Design review of the part built by this model. Coordinates are the model's own, in mm. Round coordinates to 2 decimals unless told otherwise and drop trailing zeros. Order: outer loops, then holes, each group sorted by start corner. A loop starts at its lowest first (then second) coordinate and runs counter-clockwise, first axis right, second up.
from build123d import *

# Parameters (mm, degrees)
BOSS_EXTRUDE1_DEPTH = 15
FILLET1_R           = 10
FILLET2_R           = 10


with BuildPart() as part:
    # Sketch1 → Boss-Extrude1 (new body)
    with BuildSketch(Plane(origin=(0, 0, 0), x_dir=(0, 0, -1), z_dir=(1, 0, 0))):
        with BuildLine():
            Line((-62.5, 25), (-62.5, -87.5))
            Line((-62.5, -87.5), (62.5, -87.5))
            Line((62.5, -87.5), (62.5, 25))
            ThreePointArc((62.5, 25), (106.694173824, 131.694173824), (0, 87.5))
            ThreePointArc((0, 87.5), (-106.694173824, 131.694173824), (-62.5, 25))
        make_face()
    extrude(amount=BOSS_EXTRUDE1_DEPTH)

    # Fillet1
    fillet1_edges = [part.edges().sort_by_distance(p)[0] for p in [
        (7.5, 87.5, 0),
    ]]
    fillet(fillet1_edges, radius=FILLET1_R)

    # Fillet2
    fillet2_edges = [part.edges().sort_by_distance(p)[0] for p in [
        (7.5, -87.5, -62.5),
        (7.5, -87.5, 62.5),
    ]]
    fillet(fillet2_edges, radius=FILLET2_R)


solid = part.part
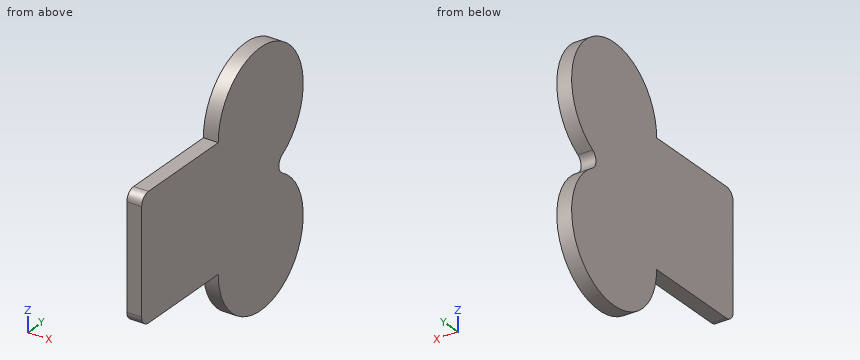
1) Take a section at C-C on z = 30.5. Give the boundary of the cut face in (x, y).
Results:
outline: (0, -87.5) - (15, -87.5) - (15, 141.19) - (0, 141.19) - close
2) To check wall thickness, follow line 1 along Z through (x, y) = (1, 85.5); line 2 along Z through (x, y) = (12, 137.5); line 3 along Z through (x, y) = (1.75, -22.5). State the ranges of each line that lie inside material, in increasing order.
Results:
line 1: z = -124.97 to 124.97
line 2: z = -100 to -25, 25 to 100
line 3: z = -62.5 to 62.5
3) Clearance check with flat-ended pins moving along their axes: P1, Ø5, axis at x = 8, z = -3, coming from the +Y side; P2, Ø1.5, axis at x = 6.5, z = -22, coming from the +Y side; P3, Ø4, axis at x = 6, y = -13, coming from the -Z side. State where each tip first meets the part, or that it passes through.
Results:
P1: stops at y = 115.89
P2: stops at y = 135.73
P3: stops at z = -62.5
4) Take a section at A-A on y = 131.5. Give the boundary of the cut face in (x, z).
Results:
outline: (0, -106.89) - (15, -106.89) - (15, -18.11) - (0, -18.11) - close; (0, 18.11) - (15, 18.11) - (15, 106.89) - (0, 106.89) - close
5) Take a section at B-B on y = -7.5. Give the boundary of the cut face in (x, z).
Results:
outline: (0, -62.5) - (15, -62.5) - (15, 62.5) - (0, 62.5) - close
